Source: CAD feature listing. Evaluate the final solid. Frame: model axes, mm. A direction names the side the tool comes from. Give positions to 0.01 mm unless a question says otherwise; leave off trailing zeros. Order: outer loops, then holes, each group sorted by start corner. A loop starts at its lowest first (then second) coordinate and runs counter-clockwise, first axis right, second up.
from build123d import *

# Parameters (mm, degrees)
SKETCH1_W           = 114.3
SKETCH1_H           = 177.8
SKETCH1_W_2         = 101.6
SKETCH1_H_2         = 165.1
BOSS_EXTRUDE1_DEPTH = 4.7625
SKETCH2_W           = 12.38677804
SKETCH2_H           = 4.7625
SKETCH2_W_2         = 12.7
BOSS_EXTRUDE2_DEPTH = 4.7625
SKETCH3_W           = 12.7
SKETCH3_H           = 4.7625
BOSS_EXTRUDE3_DEPTH = 4.7625
SKETCH4_W           = 9.525
SKETCH4_H           = 177.8
SKETCH4_W_2         = 3.81
SKETCH4_H_2         = 127
BOSS_EXTRUDE4_DEPTH = 4.7625
FILLET1_R           = 1.905


with BuildPart() as part:
    # Sketch1 → Boss-Extrude1 (new body)
    with BuildSketch(Plane(origin=(0, 0, 0), x_dir=(1, 0, 0), z_dir=(0, 1, 0))):
        Rectangle(SKETCH1_W, SKETCH1_H)
        Rectangle(SKETCH1_W_2, SKETCH1_H_2, mode=Mode.SUBTRACT)
    extrude(amount=BOSS_EXTRUDE1_DEPTH)

    # Sketch2 → Boss-Extrude2 (add)
    with BuildSketch(Plane.XY.offset(88.9)):
        with Locations((-38.1, 2.38125)):
            Rectangle(SKETCH2_W, SKETCH2_H)
        with Locations((12.7, 2.38125)):
            Rectangle(SKETCH2_W_2, SKETCH2_H)
    extrude(amount=BOSS_EXTRUDE2_DEPTH)

    # Sketch3 → Boss-Extrude3 (add)
    with BuildSketch(Plane(origin=(0, 0, -88.9), x_dir=(-1, 0, 0), z_dir=(0, 0, -1))):
        with Locations((-38.1, 2.38125)):
            Rectangle(SKETCH3_W, SKETCH3_H)
        with Locations((12.7, 2.38125)):
            Rectangle(SKETCH3_W, SKETCH3_H)
    extrude(amount=BOSS_EXTRUDE3_DEPTH)

    # Sketch4 → Boss-Extrude4 (add)
    # profile 1 of 2: a face of its own
    with BuildSketch(Plane(origin=(0, 4.7625, 0), x_dir=(-1, 0, 0), z_dir=(0, 1, 0))):
        with Locations((9.906, 0)):
            Rectangle(SKETCH4_W, SKETCH4_H)
        with Locations((9.906, 0)):
            Rectangle(SKETCH4_W_2, SKETCH4_H_2, mode=Mode.SUBTRACT)
    # profile 2 of 2: a face of its own
    with BuildSketch(Plane(origin=(0, 4.7625, 0), x_dir=(-1, 0, 0), z_dir=(0, 1, 0))):
        with Locations((-9.906, 0)):
            Rectangle(SKETCH4_W, SKETCH4_H)
        with Locations((-9.906, 0)):
            Rectangle(SKETCH4_W_2, SKETCH4_H_2, mode=Mode.SUBTRACT)
    extrude(amount=-BOSS_EXTRUDE4_DEPTH)

    # Fillet1
    fillet1_edges = [part.edges().sort_by_distance(p)[0] for p in [
        (-8.001, 2.38125, -63.5),
        (-11.811, 2.38125, -63.5),
        (8.001, 2.38125, -63.5),
        (11.811, 2.38125, -63.5),
        (-8.001, 2.38125, 63.5),
        (-11.811, 2.38125, 63.5),
        (8.001, 2.38125, 63.5),
        (11.811, 2.38125, 63.5),
        (-5.1435, 2.38125, 82.55),
        (5.1435, 2.38125, 82.55),
        (-5.1435, 2.38125, -82.55),
        (5.1435, 2.38125, -82.55),
        (-14.6685, 2.38125, -82.55),
        (-50.8, 2.38125, -82.55),
        (-50.8, 2.38125, 82.55),
        (-14.6685, 2.38125, 82.55),
        (14.6685, 2.38125, 82.55),
        (50.8, 2.38125, 82.55),
        (14.6685, 2.38125, -82.55),
        (50.8, 2.38125, -82.55),
    ]]
    fillet(fillet1_edges, radius=FILLET1_R - 0.0001)  # a hair under: the kernel refuses the full size


solid = part.part
(1) Section D-D, the plane y = 3. Count the separate pieces of the cut face and the enclosed holes in it, plus the area to 3 significant figures.
(2) Pin query (flat end, axial travel): pin 1 Ø1.5 at (x, y) = (-32, 2.5) entering from -Z; pin 2 Ø1.4 at (y, z) = (2, -92.5) entering from -X; pin 3 Ø4 at (x, z) = (-18.5, -5.5) entering from +Y; pin 4 Ø1.4 at (y, z) = (1.5, 92) entering from +X. Return the tip coordinate at first contact, or that it passes through.
(3) Line query: line 1 along X through (y, z) = (0.45, 0); line 2 along X through (y, z) = (4.3, 73); line 3 along Z through (x, y) = (-33.5, 3.4). Output: solid intervals per line, ascending.
(4) Access query for faces 4 (the flat face through (-51, 2, 88.9)), 5 (the flat face through (-13, 2, 88.9)), 6 (the flat face through (19.05, 2, 91)). Directions: +Z, -Z, +X, -X, +Y, -Y. A direction counts if a zero-diameter tool reaches every point of the face in a straight line with its end or side. Return the directions, or none.
(5) Draft query along Z for faces 1 (the flat face through (-5.144, 2, -1)), 2 (the flat face through (-14, 0, -22)), 3 (the flat face through (-38, 2, -88.9)). Return one class per face: +Z half, -Z half, draft (parallel to the pull), parting line (faces both ways), or undercut.
(6) Section C-C, the plane x = 29.5. Return loops of the section in (y, z), plus the area to 3 significant figures.
(7) Section A-A, the plane z = 36. Return loops of the section in (x, y).
(8) Section B-B, the plane z = 76. Return loops of the section in (x, y), plus the area to 3 significant figures.
Checks:
1. separate pieces: 1
1. enclosed holes: 5
1. area: 5,980 mm2
2. pin 1: stops at z = -88.9
2. pin 2: stops at x = -19.05
2. pin 3: passes through
2. pin 4: stops at x = 19.05
3. line 1: x = -57.15 to -50.8, -14.67 to -11.81, -8 to -5.14, 5.14 to 8, 11.81 to 14.67, 50.8 to 57.15
3. line 2: x = -57.15 to -50.8, -14.67 to -5.14, 5.14 to 14.67, 50.8 to 57.15
3. line 3: z = -88.9 to -82.55, 82.55 to 93.66
4. face 4: +Z, -X, +Y, -Y
4. face 5: +Z, +Y, -Y
4. face 6: +Z, +X, +Y, -Y
5. face 1: undercut
5. face 2: draft
5. face 3: -Z half
6. outline: (0, -88.9) - (4.76, -88.9) - (4.76, -82.55) - (0, -82.55) - close; (0, 82.55) - (4.76, 82.55) - (4.76, 88.9) - (0, 88.9) - close
6. area: 60.5 mm2
7. outline: (-57.15, 0) - (-50.8, 0) - (-50.8, 4.76) - (-57.15, 4.76) - close; (-14.67, 0) - (-11.81, 0) - (-11.81, 4.76) - (-14.67, 4.76) - close; (-8, 0) - (-5.14, 0) - (-5.14, 4.76) - (-8, 4.76) - close; (5.14, 0) - (8, 0) - (8, 4.76) - (5.14, 4.76) - close; (11.81, 0) - (14.67, 0) - (14.67, 4.76) - (11.81, 4.76) - close; (50.8, 0) - (57.15, 0) - (57.15, 4.76) - (50.8, 4.76) - close
8. outline: (-57.15, 0) - (-50.8, 0) - (-50.8, 4.76) - (-57.15, 4.76) - close; (-14.67, 0) - (-5.14, 0) - (-5.14, 4.76) - (-14.67, 4.76) - close; (5.14, 0) - (14.67, 0) - (14.67, 4.76) - (5.14, 4.76) - close; (50.8, 0) - (57.15, 0) - (57.15, 4.76) - (50.8, 4.76) - close
8. area: 151 mm2
